Check sheet for the modelled part. Datum: model origin and axes. Units: mm. A direction names the side the tool comes from. Coordinates: 2 decimals unless noted, no trailing zeros. Loops run counter-clockwise (first coordinate to the right, second up) from the corner with the lowest first, then second, coordinate; pieces in that order, holes last. Notation, with made-up numbers: M -26.75,1 L -2.75,1 A11 cw -2.75,22 Z; hole C 31,87.5 d5. An arc over 180 degrees is marked long. Answer in a Markdown table with one row per item. Add a question column.
Autodesk Fusion 360 part; units mm, degrees
sketch "Esboço1" plane through (0, 0, 0) normal (0, 0, 1) x (1, 0, 0)
  line L0 (0, 0) -> (110, 0)
  line L1 (110, 0) -> (110, -5)
  line L2 (55, -20) -> (5, -20)
  line L3 (0, -5) -> (0, 0)
  line L4 (0, 0) -> (55, 0)
  line L5 (0, -5) -> (0, 0)
  line L6 (35, 0) -> (75, 0)
  line L7 (0, 0) -> (10, 0)
  line L8 (10, 0) -> (10, -10)
  line L9 (0, -5) -> (0, 0)
  line L10 (10, 0) -> (50, 0)
  line L11 (50, 0) -> (50, -17)
  line L12 (50, -17) -> (10, -17)
  line L13 (10, -17) -> (10, 0)
  line L14 (10, 0) -> (50, 0)
  line L15 (50, 0) -> (50, -17)
  line L16 (50, -17) -> (10, -17)
  line L17 (10, -17) -> (10, 0)
  circle A0 centre (46.5001, -2.9491) radius 2
  circle A1 centre (46.5001, -14.1881) radius 2
  circle A2 centre (30, -14.1881) radius 2
  line L18 (30, -12.1881) -> (30, -17)
  circle A3 centre (13.4999, -14.1881) radius 2
  line L19 (0, 0) -> (5, 0)
  line L20 (0, -5) -> (0, 0)
  line L21 (110, 0) -> (105, 0)
  line L22 (110, -5) -> (110, 0)
  line L23 (55, -20) -> (110, -5)
  line L24 (5, -20) -> (0, -5)
  line L25 (0, 0) -> (5, 0)
  line L26 (5, 0) -> (5, 5)
  line L27 (5, 5) -> (0, 5)
  line L28 (0, 5) -> (0, 0)
  line L29 (105, 0) -> (110, 0)
  line L30 (110, 0) -> (110, 5)
  line L31 (110, 5) -> (105, 5)
  line L32 (105, 5) -> (105, 0)
  dimension "d1" = 110
  dimension "d3" = 55
  dimension "d5" = 40
  dimension "d7" = 40
  dimension "d8" = 17
  dimension "d9" = 40
  dimension "d10" = 17
  dimension "d11" = 4
  dimension "d12" = 4
  dimension "d13" = 4
  dimension "d14" = 5
  dimension "d15" = 5
  dimension "d16" = 5
  dimension "d17" = 5
extrude "Extrusão1" add sketch "Esboço1" along normal blind 2 contours L0 L4 L6 L8 L10 L11 L12 L13 L14 L15 L16 L17
extrude "Extrusão2" add sketch "Esboço1" along normal blind 4 contours L0 L1 L2 L3 L4 L5 L6 L7 L8 L9 L11 L12 L13 L15 L16 L17 L19 L20 L21 L22 L23 L24 L25 L29
extrude "Extrusão3" add sketch "Esboço1" along normal blind 1 contours L0 L21 L29 L30 L31 L32
extrude "Extrusão4" add sketch "Esboço1" along normal blind 1 contours L0 L4 L7 L19 L25 L26 L27 L28
sketch "Esboço2" plane through (0, 5, 0) normal (0, 1, 0) x (-1, 0, 0)
  line L0 (-110, 0) -> (-105, 0)
  line L1 (-105, 0) -> (-105, 1)
  line L2 (-105, 1) -> (-110, 1)
  line L3 (-110, 1) -> (-110, 0)
  circle A0 centre (-105, 2) radius 1
  circle A1 centre (-5, 2) radius 1
  dimension "d26" = 2
hole "Furo1" at (105, 5, 2) direction (0, -1, 0) diameter 2 depth 38 tip angle 118
hole "Furo2" at (5, 5, 2) direction (0, -1, 0) diameter 2 depth 38 tip angle 118
sketch "Esboço3" plane through (0, 0, 0) normal (0, 0, 1) x (1, 0, 0)
  line L0 (0, 0) -> (10, 0)
  line L1 (10, 0) -> (10, -2)
  line L2 (10, -2) -> (0, -2)
  line L3 (0, -2) -> (0, 0)
  line L4 (7, 0) -> (10, 0)
  line L5 (10, 0) -> (10, -20)
  line L6 (10, -20) -> (7, -20)
  line L7 (7, -20) -> (7, 0)
  line L8 (10, -20) -> (7, -20)
  line L9 (7, -20) -> (7, -2)
  line L10 (7, -2) -> (10, -2)
  line L11 (10, -2) -> (10, -20)
  line L12 (7, -20) -> (5, -20)
  line L13 (5, -20) -> (5, -2)
  line L14 (5, -2) -> (7, -2)
  line L15 (7, -2) -> (7, -20)
  dimension "d33" = 2
sketch "Esboço4" plane through (0, 0, 0) normal (0, 0, 1) x (1, 0, 0)
  line L0 (8, 0) -> (10, 0)
  line L1 (10, 0) -> (10, -20)
  line L2 (10, -20) -> (8, -20)
  line L3 (8, -20) -> (8, 0)
  line L4 (10, 0) -> (0, 0)
  line L5 (0, 0) -> (0, -2)
  line L6 (0, -2) -> (10, -2)
  line L7 (10, -2) -> (10, 0)
  line L8 (8, -20) -> (0, -20)
  line L9 (0, -20) -> (0, -2)
  line L10 (0, -2) -> (8, -2)
  line L11 (8, -2) -> (8, -20)
extrude "Extrusão6" cut sketch "Esboço4" along normal blind 2 contours L3 L6 L8 L9 L10 L11
extrude "Extrusão7" cut sketch "Esboço4" along normal blind 4 contours L3 L6 L8 L9 L10 L11
sketch "Esboço5" plane through (0, 0, 0) normal (0, 0, 1) x (1, 0, 0)
  line L0 (52, -20) -> (110, -20)
  line L1 (110, -20) -> (110, -2)
  line L2 (110, -2) -> (52, -2)
  line L3 (52, -2) -> (52, -20)
extrude "Extrusão8" cut sketch "Esboço5" along normal blind 4
extrude "Extrusão9" cut 1 faces at (108.3333, 1.6667, 1) along direction (0, 0, -1) blind 1
extrude "Extrusão10" cut 1 faces at (1.6667, 3.3333, 1) along direction (0, 0, -1) blind 1
sketch "Esboço6" plane through (0, 0, 0) normal (0, 0, 1) x (1, 0, 0)
  circle A0 centre (13.4999, -2.9491) radius 2
  point P0 (13.4999, -14.1881)
  point P1 (46.5001, -2.9491)
  dimension "d46" = 4
extrude "Extrusão14" cut sketch "Esboço6" along normal blind 2
sketch "Esboço7" plane through (0, 0, 0) normal (0, 0, 1) x (1, 0, 0)
  circle A0 centre (27.9799, -2.9491) radius 2
  point P0 (13.4999, -2.9491)
  dimension "d55" = 4
extrude "Extrusão15" cut sketch "Esboço7" along normal blind 2
extrude "Extrusão16" add sketch "Esboço1" along normal blind 2 contours A2 L18 | A1 picked at (30.6397, -14.0003)
extrude "Extrusão17" add sketch "Esboço1" along normal blind 2 contours A2 L18 picked at (30.6397, -14.0003)
Q1. Cross-section at B-B (y = -9.5). Record the cut outline in (x, z), plus the area to 3 significant figures.
Q2. Thickness scan on L1, parallel to X at y = -3.5, z = 3.05; L2, parallel to Z at x = 5, y = -0.45; L3, parallel to X at y = -13, z = 0.6. Record the ranges inside material, lowest first.
Q3. Go/stop test with flat-tipped pins: pin 1 (1.6 mm diameter, centred on y = -13.5, z = 1.5, fed in from -X); pin 2 (1.5 mm diameter, centred on y = -8.5, z = 1.5, fed in from +X); pin 3 (2 mm diameter, centred on x = 3.5, z = 2.5, fed in from -Y); pin 4 (3.5 mm diameter, centred on x = 13.5, y = -2.95, fed in from +Z). Record where each tip stops, or that it passes through.
Q4. Cross-section at D-D (y = -18). Record the cut outline in (x, z).
Q5. Cross-section at A-A (x = 5). Record the cut outline in (y, z), plus the area to 3 significant figures.
Q6. Mould release check, pull along Z, two halves, no side actions. Record for faces 1 (the face through (30, -8, 2)), 2 (the face through (4.324, -1.014, 1.263)), 3 (the face through (30, -17, 3)): released by +Z, released by -Z, zero draft, split by the parting line, or undercut.
Q7. Access from +Z, -Z, +X, -X, +Y, -Y to the whole of each face (thin tool, end or side, straight path). Record for faces 4 (the face through (10, -8, 3)), 5 (the face through (3.9, -2, 1.5)), 6 (the face through (106, -1, 2)), 7 (the face through (30, -14, 1)).
Q8. Cross-section at C-C (x = 77.5). Record the cut outline in (y, z), plus the area to 3 significant figures.
Answer key:
| question | item | result |
|---|---|---|
| 1 | outline | M 8,0 L 52,0 L 52,4 L 50,4 L 50,2 L 10,2 L 10,4 L 8,4 Z |
| 1 | area | 96.0 mm^2 |
| 2 | L1 | 8 to 10, 50 to 52 |
| 2 | L2 | 0 to 1, 3 to 4 |
| 2 | L3 | 8 to 11.89, 15.11 to 28.39, 30 to 52 |
| 3 | pin 1 | x = 8 |
| 3 | pin 2 | x = 52 |
| 3 | pin 3 | y = -2 |
| 3 | pin 4 | through |
| 4 | outline | M 8,0 L 52,0 L 52,4 L 8,4 Z |
| 5 | outline | M -2,0 L 0,0 L 0,1 L -2,1 Z; M -2,3 L 0,3 L 0,4 L -2,4 Z |
| 5 | area | 4.00 mm^2 |
| 6 | face 1 | released by +Z |
| 6 | face 2 | undercut |
| 6 | face 3 | zero draft |
| 7 | face 4 | +Z, +Y |
| 7 | face 5 | +Z, -Z, -X, -Y |
| 7 | face 6 | +Y, -Y |
| 7 | face 7 | +Z, -Z |
| 8 | outline | M -2,0 L 0,0 L 0,4 L -2,4 Z |
| 8 | area | 8.00 mm^2 |
